```python
from build123d import *

# Parameters (mm, degrees)
SKETCH_1_W             = 295
SKETCH_1_H             = 91.45
EXTRUDE_1_DEPTH        = 3
SKETCH_4_W             = 3
SKETCH_4_H             = 91.45
EXTRUDE_2_DEPTH        = 104
SKETCH_5_W             = 70
SKETCH_5_H             = 91.45
EXTRUDE_3_DEPTH        = 3
CUT_EXTRUDE_1_DEPTH    = 322.574228766
HOLE_WIZARD_M6_1_D     = 6.6
HOLE_WIZARD_M6_1_DEPTH = 3
HOLE_WIZARD_M3_1_D     = 3.4
SKETCH_39_W            = 3
SKETCH_39_H            = 51.410454545
EXTRUDE_5_DEPTH        = 10
SKETCH_42_W            = 3
SKETCH_42_H            = 51.410454545
EXTRUDE_6_DEPTH        = 117
CUT_EXTRUDE_5_REACH    = 219.563
SKETCH_44_W            = 114
SKETCH_44_H            = 52.54090909


with BuildPart() as part:
    # ｽｹｯﾁ1 → ﾎﾞｽ - 押し出し1 (new body)
    with BuildSketch(Plane.XY):
        with Locations((28.42242268, -19.734793814)):
            Rectangle(SKETCH_1_W, SKETCH_1_H)
    extrude(amount=EXTRUDE_1_DEPTH)

    # ｽｹｯﾁ4 → ﾎﾞｽ - 押し出し2 (add)
    with BuildSketch(Plane.XY.offset(3)):
        with Locations((-117.57757732, -19.734793814)):
            Rectangle(SKETCH_4_W, SKETCH_4_H)
        with Locations((174.42242268, -19.734793814)):
            Rectangle(SKETCH_4_W, SKETCH_4_H)
    extrude(amount=EXTRUDE_2_DEPTH)

    # ｽｹｯﾁ5 → ﾎﾞｽ - 押し出し3 (add)
    with BuildSketch(Plane.XY.offset(107)):
        with Locations((-84.07757732, -19.734793814)):
            Rectangle(SKETCH_5_W, SKETCH_5_H)
        with Locations((140.92242268, -19.734793814)):
            Rectangle(SKETCH_5_W, SKETCH_5_H)
    extrude(amount=EXTRUDE_3_DEPTH)

    # ｽｹｯﾁ24 → ｶｯﾄ - 押し出し1 (cut, through all)
    with BuildSketch(Plane(origin=(175.92242268, 0, 0), x_dir=(0, 0, -1), z_dir=(1, 0, 0))):
        Polygon((-110, 25.990206186), (0, -14.009793814), (0, 25.990206186), align=None)
        Polygon((-110, -65.459793814), (0, -65.459793814), (-110, -24.009793814), align=None)
    extrude(amount=-CUT_EXTRUDE_1_DEPTH, mode=Mode.SUBTRACT)

    # M6 すきま穴1
    with Locations(Plane.XY.offset(110)):
        with Locations((113.92242268, 13.990206186), (113.92242268, -11.009793814), (138.92242268, -11.009793814), (138.92242268, 13.990206186), (-57.07757732, 13.990206186), (-57.07757732, -11.009793814), (-82.07757732, -11.009793814), (-82.07757732, 13.990206186)):
            Hole(HOLE_WIZARD_M6_1_D / 2, depth=HOLE_WIZARD_M6_1_DEPTH)

    # M3 すきま穴1 (through all)
    with Locations(Plane.XY.offset(3)):
        with Locations((-72.57757732, -33.418884724), (-81.57757732, -40.418884724), (-49.57757732, -50.918884724), (138.42242268, -40.418884724), (129.42242268, -33.418884724), (112.92242268, -50.918884724)):
            Hole(HOLE_WIZARD_M3_1_D / 2)

    # ｽｹｯﾁ39 → ﾎﾞｽ - 押し出し5 (add)
    with BuildSketch(Plane.XY.offset(3)):
        with Locations((-30.07757732, -38.624111997)):
            Rectangle(SKETCH_39_W, SKETCH_39_H)
        with Locations((86.92242268, -38.624111997)):
            Rectangle(SKETCH_39_W, SKETCH_39_H)
    extrude(amount=EXTRUDE_5_DEPTH)

    # ｽｹｯﾁ42 → ﾎﾞｽ - 押し出し6 (add)
    with BuildSketch(Plane(origin=(88.42242268, 0, 0), x_dir=(0, 0, -1), z_dir=(1, 0, 0))):
        with Locations((-11.5, -38.624111997)):
            Rectangle(SKETCH_42_W, SKETCH_42_H)
    extrude(amount=-EXTRUDE_6_DEPTH)

    # ｽｹｯﾁ44 → ｶｯﾄ - 押し出し5 (cut, up to next)
    with BuildSketch(Plane(origin=(0, 0, 0), x_dir=(-1, 0, 0), z_dir=(0, 0, -1)), mode=Mode.PRIVATE) as cut_extrude_5_sk1:
        with Locations((-28.42242268, -39.189339269)):
            Rectangle(SKETCH_44_W, SKETCH_44_H)
    cut_extrude_5_tool1 = extrude(cut_extrude_5_sk1.sketch, amount=-CUT_EXTRUDE_5_REACH, mode=Mode.PRIVATE) & part.part
    add(cut_extrude_5_tool1.solids().sort_by_distance((28.422423, -39.189339, 0))[0], mode=Mode.SUBTRACT)


solid = part.part
```
Here's how the part is built. I have some questions about the finished solid (model axes, mm). A direction names the side the tool comes from. Round coordinates to 2 decimals unless told otherwise and drop trailing zeros. Write each loop counter-clockwise with the first axis right and the second up, starting at its lowest first coordinate (ties: lowest second). Pieces come first, ordered by that corner, then holes. Notation, with made-up numbers: M 16,-17.75 L 75,-17.75 A22 cw 75,18.25 Z; hole C 0.25,-20.75 d1. An arc over 180 degrees is marked long. Answer as CSV lines item,"result". Start each with the question number.
1. Thinking about a two-plate mould opening in Z: for faces 1 (the flat face through (130, -38, 3)), 2 (the flat face through (-31.578, -39, 8)), 3 (the flat face through (139, 0, 107)), 4 (the flat face through (-117.19, 4.6, 51.18)), which applies, released by +Z, released by -Z, zero draft, split by the parting line, or undercut?
2. I need wall thicknesses on probe 1 along X at (y, z) = (-26, 82); probe 2 along X at (y, z) = (-34, 10.5); probe 3 along Z at (x, y) = (143, -28). Which ranges of each line are inside material? Lowest first, please.
3. Suppose I cut it at D-D on y = 8. Write out the boundary of the cut face in (x, z), then the cut area to 3 significant figures.
4. Suppose I cut it at C-C on x = -56.5. Write out the boundary of the cut face in (y, z), then the cut area to 3 significant figures.
5. On a 3-axis mill with a long thin cutter (end or side, diameter ignored), from which of +Z, -Z, +X, -X, +Y, -Y can I reach the whole of each face in a straight line? I mean faces 5 (the flat face through (88.422, -39, 8)), 6 (the flat face through (172.922, -20, 54)), 7 (the flat face through (24, -12.919, 11)). Say none if no direction works.
6. Suppose I cut it at A-A on y = -17. Write out the boundary of the cut face in (x, z), then the cut area to 3 significant figures.
7. I'm going to push flat-ended pins straight in: pin 1 Ø4 at (x, y) = (-82.08, -11.01) entering from +Z; pin 2 Ø7.5 at (x, y) = (113.92, 13.99) entering from +Z; pin 3 Ø2.5 at (x, y) = (-49.58, -50.92) entering from -Z. Where does each tip first touch, or does it pass through?
8. Suppose I cut it at B-B on z = 100. Write out the boundary of the cut face in (x, y).
Check result:
1,face 1,"undercut"
1,face 2,"zero draft"
1,face 3,"undercut"
1,face 4,"released by -Z"
2,probe 1,"x = -119.08 to -116.08, 172.92 to 175.92"
2,probe 2,"x = -119.08 to -116.08, -31.58 to 88.42, 172.92 to 175.92"
2,probe 3,"z = 0 to 3"
3,outline,"M -119.08,60.53 L -116.08,60.53 L -116.08,107 L -49.08,107 L -49.08,110 L -119.08,110 Z; M 105.92,107 L 172.92,107 L 172.92,60.53 L 175.92,60.53 L 175.92,110 L 105.92,110 Z"
3,area,"699 mm2"
4,outline,"M -65.46,0 L -14.01,0 L -12.92,3 L -64.33,3 Z; M -25.14,107 L -14.26,107 L -14.26,110 L -24.01,110 Z; M -7.76,107 L 10.74,107 L 10.74,110 L -7.76,110 Z; M 17.24,107 L 24.9,107 L 25.99,110 L 17.24,110 Z"
4,area,"265 mm2"
5,face 5,"+Z, +Y, -Y"
5,face 6,"+Y, -Y"
5,face 7,"+Z, -Z, +Y"
6,outline,"M -119.08,0 L -28.58,0 L -28.58,10 L 85.42,10 L 85.42,0 L 175.92,0 L 175.92,110 L 105.92,110 L 105.92,107 L 172.92,107 L 172.92,3 L 88.42,3 L 88.42,13 L -31.58,13 L -31.58,3 L -116.08,3 L -116.08,107 L -49.08,107 L -49.08,110 L -119.08,110 Z"
6,area,"1,990 mm2"
7,pin 1,"stops at z = 3"
7,pin 2,"stops at z = 110"
7,pin 3,"passes through"
8,outline,"M -119.08,-27.78 L -116.08,-27.78 L -116.08,22.35 L -119.08,22.35 Z; M 172.92,-27.78 L 175.92,-27.78 L 175.92,22.35 L 172.92,22.35 Z"
